Verification items for the finished model (mm, model axes). Coordinates: 2 decimals unless noted, no trailing zeros. Loops run counter-clockwise (first coordinate to the right, second up) from the corner with the lowest first, then second, coordinate; pieces in that order, holes last. Notation, with made-up numbers: (68.5, 89.25) -> (82.5, 89.25) arc R20 ccw to (82.5, 98.25) -> close; hole circle Ø3 at (17, 58.5). An arc over 180 degrees is marked (long way). Answer as a JSON object with one key per item and string values. Group by question number.
Q1. Scan lines: L1, parallel to Y at x = -70, z = 1.95; L2, parallel to X at y = -80, z = 1.55; L3, parallel to Y at x = -54, z = 1. Record each from-to range of solid material in increasing order.
Q2. Cross-section at B-B on x = 55. Record the boundary of the cut face in (y, z), and give its area (3 significant figures).
Q3. Cross-section at A-A on z = 1. Record the boundary of the cut face in (x, y).
Q4. Gauge pin test, flat ends, axial feed: pin 1 Ø1.5 at (x, z) = (-58, 1.5) entering from +Y; pin 2 Ø5 at (x, y) = (70, 80) entering from -Z; pin 3 Ø0.9 at (y, z) = (120, 1) entering from +X; pin 4 Ø1.5 at (y, z) = (72, 1) entering from -X. Record the tip position at first contact, or that the pin passes through.
Autodesk Inventor part; units mm, degrees
ref_plane "YZ Plane" through (0, 0, 0) normal (1, 0, 0) x (0, 1, 0)
ref_plane "XZ Plane" through (0, 0, 0) normal (0, 1, 0) x (-1, 0, 0)
ref_plane "XY Plane" through (0, 0, 0) normal (0, 0, 1) x (1, 0, 0)
sketch "Sketch1" plane through (0, 0, 0) normal (0, 0, 1) x (1, 0, 0)
  point P0 (0, 0)
sketch "Sketch2" plane through (0, 0, 0) normal (0, 0, 1) x (1, 0, 0)
  line L0 (94.9998, -95.0001) -> (-94.9998, -95.0001)
  line L1 (-94.9998, -95.0001) -> (-94.9998, 95.0001)
  line L2 (-94.9998, 95.0001) -> (94.9998, 95.0001)
  line L3 (94.9998, 95.0001) -> (94.9998, -95.0001)
  line L4 (94.9998, -95.0001) -> (-94.9998, 95.0001) construction
  line L5 (-94.9998, -95.0001) -> (94.9998, 95.0001) construction
  line L6 (-36.0001, 94.9999) -> (36.0001, 94.9999)
  line L7 (36.0001, 94.9999) -> (36.0001, 135.0001)
  line L8 (36.0001, 135.0001) -> (-36.0001, 135.0001)
  line L9 (-36.0001, 135.0001) -> (-36.0001, 94.9999)
  line L10 (-36.0001, 94.9999) -> (36.0001, 135.0001) construction
  line L11 (36.0001, 94.9999) -> (-36.0001, 135.0001) construction
  point P0 (0, 115)
  point P1 (-36.0001, 95.0001)
  point P2 (36.0001, 95.0001)
extrude "Extrusion1" add sketch "Sketch2" along normal blind 3
sketch "Standoff holes" plane through (0, 0, 3) normal (0, 0, 1) x (1, 0, 0)
  circle A0 centre (70, 80) radius 1.5001
  circle A1 centre (70, -80) radius 1.5001
  circle A2 centre (-70, 80) radius 1.5001
  circle A3 centre (-70, -80) radius 1.5001
extrude "Extrusion2" cut sketch "Standoff holes" against normal blind 3
fillet "Fillet5" radius 25 4 edges at (-94.9998, 95.0001, 1.5) (94.9998, 95.0001, 1.5) (-94.9998, -95.0001, 1.5) (94.9998, -95.0001, 1.5)
fillet "Fillet6" radius 5 2 edges at (-36.0001, 135.0001, 1.5) (36.0001, 135.0001, 1.5)
sketch "Large Hammond mount holes" plane through (0, 0, 3) normal (0, 0, 1) x (1, 0, 0)
  circle A0 centre (17.6939, 39.717) radius 2.0002
  circle A1 centre (-18.3061, 125.717) radius 2.0002
sketch "BNC flange mount" plane through (0, 0, 3) normal (0, 0, 1) x (1, 0, 0)
  circle A0 centre (0, 0) radius 6.5
sketch "PX4FLOW mount holes" plane through (0, 0, 0) normal (0, 0, -1) x (-1, 0, 0)
  circle A0 centre (19.5263, 119.2212) radius 1.5872
  circle A1 centre (-4.2863, 119.2212) radius 1.5872
  circle A2 centre (-4.2863, 119.2212) radius 1.5872
  circle A3 centre (-4.2863, 89.0588) radius 1.5872
  circle A4 centre (19.5263, 89.0588) radius 1.5872
sketch "Guard rails mount holes" plane through (0, 0, 0) normal (0, 0, -1) x (-1, 0, 0)
  circle A0 centre (-32.3501, 38.3605) radius 1.2501
  circle A1 centre (-38.3605, 32.3501) radius 1.2501
  circle A2 centre (-60.6344, 66.6448) radius 1.2501
  circle A3 centre (-66.6448, 60.6344) radius 1.2501
  circle A4 centre (-38.3605, -32.3501) radius 1.2501
  circle A5 centre (-32.3501, -38.3605) radius 1.2501
  circle A6 centre (-66.6448, -60.6344) radius 1.2501
  circle A7 centre (-60.6344, -66.6448) radius 1.2501
  circle A8 centre (32.3501, -38.3605) radius 1.2501
  circle A9 centre (38.3605, -32.3501) radius 1.2501
  circle A10 centre (60.6344, -66.6448) radius 1.2501
  circle A11 centre (66.6448, -60.6344) radius 1.2501
  circle A12 centre (38.3605, 32.3501) radius 1.2501
  circle A13 centre (32.3501, 38.3605) radius 1.2501
  circle A14 centre (66.6448, 60.6344) radius 1.2501
  circle A15 centre (60.6344, 66.6448) radius 1.2501
properties part number "payload_bay_square_drill_holes" material "CFRP"
Computed values:
{
 "1": {"L1": "y = -95 to -81.5, -78.5 to 78.5, 81.5 to 95", "L2": "x = -92.91 to -71.5, -68.5 to 68.5, 71.5 to 92.91", "L3": "y = -95 to 95"},
 "2": {"outline": "(-95, 0) -> (95, 0) -> (95, 3) -> (-95, 3) -> close", "area": "570 mm²"},
 "3": {"outline": "(-95, -70) arc R25 ccw to (-70, -95) -> (70, -95) arc R25 ccw to (95, -70) -> (95, 70) arc R25 ccw to (70, 95) -> (36, 95) -> (36, 130) arc R5 ccw to (31, 135) -> (-31, 135) arc R5 ccw to (-36, 130) -> (-36, 95) -> (-70, 95) arc R25 ccw to (-95, 70) -> close; hole circle Ø3 at (-70, -80); hole circle Ø3 at (-70, 80); hole circle Ø3 at (70, -80); hole circle Ø3 at (70, 80)"},
 "4": {"pin 1": "stops at y = 95", "pin 2": "stops at z = 0", "pin 3": "stops at x = 36", "pin 4": "stops at x = -94.97"}
}
